CAD build for the part. Positions are in the model's coordinates, mm. A direction names the side the tool comes from. Give positions to 0.01 mm unless a question says otherwise; leave off trailing zeros. Order: outer loops, then holes, each group sorted by start corner. A loop starts at its lowest first (then second) coordinate and runs counter-clockwise, first axis right, second up.
```python
from build123d import *

# Parameters (mm, degrees)
F0_R     = 5.5
F1_DEPTH = 10
F2_R     = 9
F2_R_2   = 5.5
F3_DEPTH = 2
F4_SIZE  = 1


with BuildPart() as f1:
    # F0 (on Top) → F1 (new body)
    with BuildSketch(Plane.XY):
        with BuildLine():
            Line((10, -6.63325), (10, 6.63325))
            ThreePointArc((10, 6.63325), (0, 12), (-10, 6.63325))
            Line((-10, 6.63325), (-10, -6.63325))
            ThreePointArc((-10, -6.63325), (0, -12), (10, -6.63325))
        make_face()
        Circle(F0_R, mode=Mode.SUBTRACT)
    extrude(amount=F1_DEPTH)

    # F2 (on face) → F3 (cut)
    with BuildSketch(Plane.XY.offset(10)):
        Circle(F2_R)
        Circle(F2_R_2, mode=Mode.SUBTRACT)
    extrude(amount=-F3_DEPTH, mode=Mode.SUBTRACT)

    # F4
    f4_edges = [f1.edges().sort_by_distance(p)[0] for p in [
        (0, -12, 10),
        (0, 12, 10),
    ]]
    chamfer(f4_edges, length=F4_SIZE)


solid = f1.part
```
Item 1: Wall check: L1, parallel to Z at x = 7, y = 2.75; L2, parallel to Y at x = 3, z = 8.5; L3, parallel to Y at x = 1.75, z = 3.5. Give the ranges that are in metal, low to high.
Item 2: Drop flat-ended pins along their axis: pin 1 Ø2 at (x, z) = (7, 2) entering from -Y; pin 2 Ø5 at (x, z) = (-5.5, 1) entering from +Y; pin 3 Ø6.5 at (x, y) = (0, 0) entering from -Z. Give the stop position or say it passes through.
Item 3: Slice it at B-B (y = 0). Give the cut face in (x, z).
Item 4: Slice it at A-A (x = 0). Give the cut face in (y, z), and give its area (3 significant figures).
Item 5: Tool access for faces 4 (the face through (-4, -4, 8)), 5 (the face through (0.2, 11.2, 9.8)): list every direction of +Z, -Z, +X, -X, +Y, -Y with a clear straight run to the whole face (end or side of a thin tool).
Item 6: Slice it at D-D (y = 3.25). Give the cut face in (x, z).
Item 7: Two-plate mould, pull along X, no slides. Class faces 1 (the face through (-1.172, 8.923, 9.014)), 2 (the face through (0, 12, 4)), 3 (the face through (-10, 0, 5)): released by +X, released by -X, zero draft, split by the parting line, or undercut.
Item 8: Slice it at C-C (z = 2.5). Give the cut face in (x, y), and give its area (3 significant figures).
A:
1. L1: z = 0 to 8
1. L2: y = -11.62 to -8.49, 8.49 to 11.62
1. L3: y = -11.87 to -5.21, 5.21 to 11.87
2. pin 1: stops at y = -10.39
2. pin 2: stops at y = 11.62
2. pin 3: passes through
3. outline: (-10, 0) - (-5.5, 0) - (-5.5, 8) - (-9, 8) - (-9, 10) - (-10, 10) - close; (5.5, 0) - (10, 0) - (10, 10) - (9, 10) - (9, 8) - (5.5, 8) - close
4. outline: (-12, 0) - (-5.5, 0) - (-5.5, 8) - (-9, 8) - (-9, 10) - (-11, 10) - (-12, 9) - close; (5.5, 0) - (12, 0) - (12, 9) - (11, 10) - (9, 10) - (9, 8) - (5.5, 8) - close
4. area: 115 mm2
5. face 4: +Z
5. face 5: +Z, +Y
6. outline: (-10, 0) - (-4.44, 0) - (-4.44, 8) - (-8.39, 8) - (-8.39, 10) - (-10, 10) - close; (4.44, 0) - (10, 0) - (10, 10) - (8.39, 10) - (8.39, 8) - (4.44, 8) - close
7. face 1: undercut
7. face 2: split by the parting line
7. face 3: released by -X
8. outline: (-10, -6.63) arc R12 ccw to (10, -6.63) - (10, 6.63) arc R12 ccw to (-10, 6.63) - close; hole circle Ø11 at (0, 0)
8. area: 321 mm2
